Verification items for the finished model (mm, model axes). A direction names the side the tool comes from. Coordinates: 2 decimals unless noted, no trailing zeros. Order: outer loops, then holes, each group sorted by start corner. A loop starts at its lowest first (then second) coordinate and runs counter-clockwise, first axis right, second up. Notation, with made-up numbers: (85.5, 11.25) -> (141.5, 11.25) arc R7 ccw to (141.5, 18.25) -> close; hole circle Ø7 at (-23, -3.5). An arc over 180 degrees is marked (long way). Write item = value, one per line. Start each with the question number.
1. Set-up check for faces 4 (the flat face through (29, 13.141, 17)), 5 (the cylindrical face through (14.051, 25.974, 13.605)), 6 (the cylindrical face through (-3.85, 52.49, 22.07)): record each of +Z, -Z, +X, -X, +Y, -Y from which the full face is reachable in a straight line by a thin tool's end or side.
2. Go/stop test with flat-tipped pins: P1, Ø1.6, axis at x = 34, z = 18, coming from the -Y side; P2, Ø3, axis at x = -4, y = 29, coming from the +Z side; P3, Ø20.5, axis at x = 27.71, y = 25.84, coming from the +Z side; P4, Ø6.5, axis at x = 8.66, y = 65.47, coming from the +Z side. Record where each tip stops, or that it passes through.
3. Cross-section at D-D on x = -34. Record the cut outline in (y, z).
4. Release check for a two-part mould opening along X. For faces 1 (the flat face through (-13, 49, 23.876)), 2 (the cylindrical face through (-23.76, 66.42, 13.605)), 3 (the cylindrical face through (-29.818, 75.736, 25.578)) record: +X half, -X half, draft (parallel to the pull), parting line (faces both ways), or undercut.
5. Thickness scan on line 1 along Y through (x, z) = (28, 17); line 2 along X through (y, z) = (22, 7); line 3 along Y through (x, z) = (32.5, 4). Record the ranges inside material, lowest first. Write a range as from..to.
6. Cross-section at C-C on y = 29. Record the cut outline in (x, z) (3 decimals), plus the area to 3 significant figures.
7. Cross-section at A-A on x = 9.5. Record the cut outline in (y, z) (3 decimals).
8. Cross-section at B-B on z = 27. Record the cut outline in (x, y) (3 decimals), plus the area to 3 significant figures.
from build123d import *

# Parameters (mm, degrees)
F0_W      = 82.55
F0_H      = 120.65
F1_DEPTH  = 12.7
F3_DEPTH  = 25.4
F5_DEPTH  = 11.3716514647
F6_W      = 44.45
F6_H      = 12.7
F7_DEPTH  = 25.4
F8_W      = 25.4
F8_H      = 25.4
F9_DEPTH  = 6.35
F10_R     = 6.35
F11_DEPTH = 19.051
F13_DEPTH = 15.748
F14_R     = 4.826
F15_DEPTH = 28.449
F16_R     = 8.001
F16_R_2   = 4.826
F17_DEPTH = 4.572
F18_W     = 12.7
F18_H     = 28.448
F19_DEPTH = 25.4
F20_R     = 3.175
F20_R_2   = 5.588
F21_DEPTH = 12.701
F22_R     = 3.175
F23_DEPTH = 25.4
F25_DEPTH = 25.4
F26_R     = 16.002
F27_R     = 3.175


with BuildPart() as f1:
    # F0 (on Top) → F1 (new body)
    with BuildSketch(Plane.XY):
        with Locations((-0.8694417775, 29.0160470424)):
            Rectangle(F0_W, F0_H)
    extrude(amount=F1_DEPTH)

    # F2 (on face) → F3 (join)
    with BuildSketch(Plane.XY.offset(12.7)):
        Polygon((-30.7727903128, 89.3410470424), (-42.1444417775, 89.3410470424), (-42.1444417775, 76.6410470424), (-42.1444417775, 38.5410470424), (-30.7727903128, 38.5410470424), (-30.7727903128, 76.6410470424), (40.4055582225, 76.6410470424), (40.4055582225, 89.3410470424), align=None)
    extrude(amount=F3_DEPTH)

    # F4 (on face) → F5 (join, through all)
    with BuildSketch(Plane.YZ.offset(-30.7727903128)):
        Polygon((38.5410470424, 12.7), (38.5410470424, 38.1), (-5.4530434699, 12.7), align=None)
    extrude(amount=-F5_DEPTH)

    # F6 (on face) → F7 (cut)
    with BuildSketch(Plane(origin=(0, 89.3410470424, 0), x_dir=(-1, 0, 0), z_dir=(0, 1, 0))):
        with Locations((0.8694417775, 31.75)):
            Rectangle(F6_W, F6_H)
    extrude(amount=-F7_DEPTH, mode=Mode.SUBTRACT)

    # F8 (on face) → F9 (join)
    with BuildSketch(Plane.XY.offset(12.7)):
        with Locations((27.7055582225, 25.8410470424)):
            Rectangle(F8_W, F8_H)
    extrude(amount=F9_DEPTH)

    # F10 (on face) → F11 (cut, through all)
    with BuildSketch(Plane.XY.offset(19.05)):
        with Locations((27.7055582225, 25.8410470424)):
            Circle(F10_R)
    extrude(amount=-F11_DEPTH, mode=Mode.SUBTRACT)

    # F12 (on face) → F13 (join)
    with BuildSketch(Plane.XY.offset(12.7)):
        with BuildLine():
            Line((-30.7727903128, 65.4650470424), (-30.7727903128, 40.0650470424))
            Line((-30.7727903128, 40.0650470424), (-16.5487903128, 40.0650470424))
            ThreePointArc((-16.5487903128, 40.0650470424), (-3.8487903128, 52.7650470424), (-16.5487903128, 65.4650470424))
            Line((-16.5487903128, 65.4650470424), (-30.7727903128, 65.4650470424))
        make_face()
    extrude(amount=F13_DEPTH)

    # F14 (on face) → F15 (cut, through all)
    with BuildSketch(Plane.XY.offset(28.448)):
        with Locations((-16.5487903128, 52.7650470424)):
            Circle(F14_R)
    extrude(amount=-F15_DEPTH, mode=Mode.SUBTRACT)

    # F16 (on face) → F17 (cut)
    with BuildSketch(Plane.XY.offset(28.448)):
        with Locations((-16.5487903128, 52.7650470424)):
            Circle(F16_R)
        with Locations((-16.5487903128, 52.7650470424)):
            Circle(F16_R_2, mode=Mode.SUBTRACT)
    extrude(amount=-F17_DEPTH, mode=Mode.SUBTRACT)

    # F18 (on face) → F19 (cut)
    with BuildSketch(Plane.XY.offset(12.7)):
        with Locations((-0.8694417775, -17.0849529576)):
            Rectangle(F18_W, F18_H)
        with BuildLine():
            ThreePointArc((5.4805582225, -2.8609529576), (-0.8694417775, 3.4890470424), (-7.2194417775, -2.8609529576))
            Line((-7.2194417775, -2.8609529576), (5.4805582225, -2.8609529576))
        make_face()
    extrude(amount=-F19_DEPTH, mode=Mode.SUBTRACT)

    # F20 (on face) → F21 (cut, through all)
    with BuildSketch(Plane.XY.offset(12.7)):
        with Locations((-18.5224417775, 19.4910470424)):
            Circle(F20_R)
        with Locations((24.4035582225, -15.3069529576)):
            Circle(F20_R_2)
        with Locations((27.7055582225, 65.4650470424)):
            Circle(F20_R_2)
        with Locations((8.6555582225, 65.4650470424)):
            Circle(F20_R_2)
    extrude(amount=-F21_DEPTH, mode=Mode.SUBTRACT)

    # F22 (on face) → F23 (cut)
    with BuildSketch(Plane.XZ.offset(-76.6410470424)):
        with Locations((30.8805582225, 25.4)):
            Circle(F22_R)
    extrude(amount=-F23_DEPTH, mode=Mode.SUBTRACT)

    # F24 (on face) → F25 (cut)
    with BuildSketch(Plane.XY.offset(12.7)):
        with BuildLine():
            Line((-42.1444417775, -31.3089529576), (-29.4444417775, -31.3089529576))
            ThreePointArc((-29.4444417775, -31.3089529576), (-33.1641856564, -22.3286968366), (-42.1444417775, -18.6089529576))
            Line((-42.1444417775, -18.6089529576), (-42.1444417775, -31.3089529576))
        make_face()
    extrude(amount=-F25_DEPTH, mode=Mode.SUBTRACT)

    # F26
    f26_edges = [f1.edges().sort_by_distance(p)[0] for p in [
        (40.405558, -31.308953, 6.35),
    ]]
    fillet(f26_edges, radius=F26_R)

    # F27
    f27_edges = [f1.edges().sort_by_distance(p)[0] for p in [
        (-30.77279, 17.306002, 12.7),
        (-30.77279, 40.065047, 20.574),
        (-23.66079, 40.065047, 12.7),
        (-30.77279, 52.765047, 28.448),
        (4.816384, 76.641047, 12.7),
        (-30.77279, 65.465047, 20.574),
        (-30.77279, 76.641047, 25.4),
        (15.005558, 13.141047, 15.875),
        (15.005558, 38.541047, 15.875),
        (-23.094442, 82.991047, 38.1),
        (40.405558, 82.991047, 38.1),
        (21.355558, 82.991047, 38.1),
        (27.705558, 13.141047, 12.7),
        (15.005558, 25.841047, 12.7),
        (27.705558, 38.541047, 12.7),
        (-23.66079, 65.465047, 12.7),
        (-3.84879, 52.765047, 12.7),
    ]]
    fillet(f27_edges, radius=F27_R)


solid = f1.part
Worked out:
q1.face_4 = +Z, +X, -Y
q1.face_5 = +Z, -Y
q1.face_6 = +Z, +X
q2.P1 = 13.14
q2.P2 = 12.7
q2.P3 = 19.05
q2.P4 = through
q3.outline = (-21.56, 0) -> (89.34, 0) -> (89.34, 38.1) -> (38.54, 38.1) -> (-5.45, 12.7) -> (-21.56, 12.7) -> close
q4.face_1 = undercut
q4.face_2 = draft
q4.face_3 = +X half
q5.line_1 = 13.14..19.5, 32.18..38.54, 76.64..89.34
q5.line_2 = -42.14..-20.47, -16.58..22.65, 32.76..40.41
q5.line_3 = -29.11..21.68, 30..62.59, 68.34..89.34
q6.outline = (-42.144, 0) -> (22.197, 0) -> (22.197, 19.05) -> (15.006, 19.05) -> (15.006, 15.875) arc R3.175 cw to (11.831, 12.7) -> (-27.598, 12.7) arc R3.175 cw to (-30.773, 15.875) -> (-30.773, 32.591) -> (-42.144, 32.591) -> close; (33.214, 0) -> (40.406, 0) -> (40.406, 19.05) -> (33.214, 19.05) -> close
q6.area = 1,230 mm²
q7.outline = (-31.309, 0) -> (59.941, 0) -> (59.941, 12.7) -> (-31.309, 12.7) -> close; (70.989, 0) -> (89.341, 0) -> (89.341, 25.4) -> (76.641, 25.4) -> (76.641, 15.875) arc R3.175 cw to (73.466, 12.7) -> (70.989, 12.7) -> close
q8.outline = (-42.144, 19.315) -> (-30.773, 19.315) -> (-30.773, 36.89) arc R3.175 cw to (-27.598, 40.065) -> (-16.549, 40.065) arc R12.7 ccw to (-16.549, 65.465) -> (-27.598, 65.465) arc R3.175 cw to (-30.773, 68.64) -> (-30.773, 73.466) arc R3.175 cw to (-27.598, 76.641) -> (-23.094, 76.641) -> (-23.094, 89.341) -> (-42.144, 89.341) -> close; (21.356, 76.641) -> (28.138, 76.641) -> (28.138, 89.341) -> (21.356, 89.341) -> close; (33.623, 76.641) -> (40.406, 76.641) -> (40.406, 89.341) -> (33.623, 89.341) -> close; hole circle Ø16.002 at (-16.549, 52.765)
q8.area = 1,490 mm²
